For this review, use the dimensioned drawing (mm, ordinates from the lowest corner) and the shaded views. A direction names the side the tool comes from. Coordinates: 2 decimals unless noted, no trailing zeros. Loops run counter-clockwise (first coordinate to the right, second up) from the corner with the lowest first, then second, coordinate; pieces in that order, holes last.
1. Take a section at D-D, the plane y = 65.5. State the section outline as (x, z) points, then the cut area to 3 significant figures.
2. Mouldability with a two-part tool opening along X and no side actions: class the marked faces 1, 2 and 3 as pulls with the +X half, pulls with the -X half, needs draft (parallel to the pull), parting line crosses it, or undercut.
3. Machinability: for the marked faces 4, 5 and 6, which of the approach directions +Z, -Z, +X, -X, +Y, -Y give a long, thin tool a straight path to every point of the face, cutting with its end or side? Answer none if there is none.
4. Take a section at C-C, the plane x = 18. State the section outline as (y, z) points, then the cut area to 4 significant figures.
5. Take a section at A-A, the plane z = 11.5. State the section outline as (x, y) points, then the cut area to 3 significant figures.
6. Take a section at B-B, the plane x = 7.5. State the section outline as (y, z) points.
7. Clearance check with flat-ended pins moving along their axes: P1, Ø15, axis at x = 16.5, y = 123.5, coming from the -Z side; P2, Ø20, axis at x = 16, z = 6.5, coming from the +Y side; P3, Ø10, axis at y = 170.5, z = 44, coming from the -X side; P4, Ø4.5, axis at x = 32, z = 41.5, coming from the -Y side. State where each tip first meets the part, or that it passes through.
8. To check wall thickness, follow probe 1 along Z at (x, y) = (29, 45.5); probe 2 along Y at (x, z) = (18, 7.5); probe 3 along Y at (x, z) = (43, 44). State the ranges of each line that lie inside material, in increasing order.
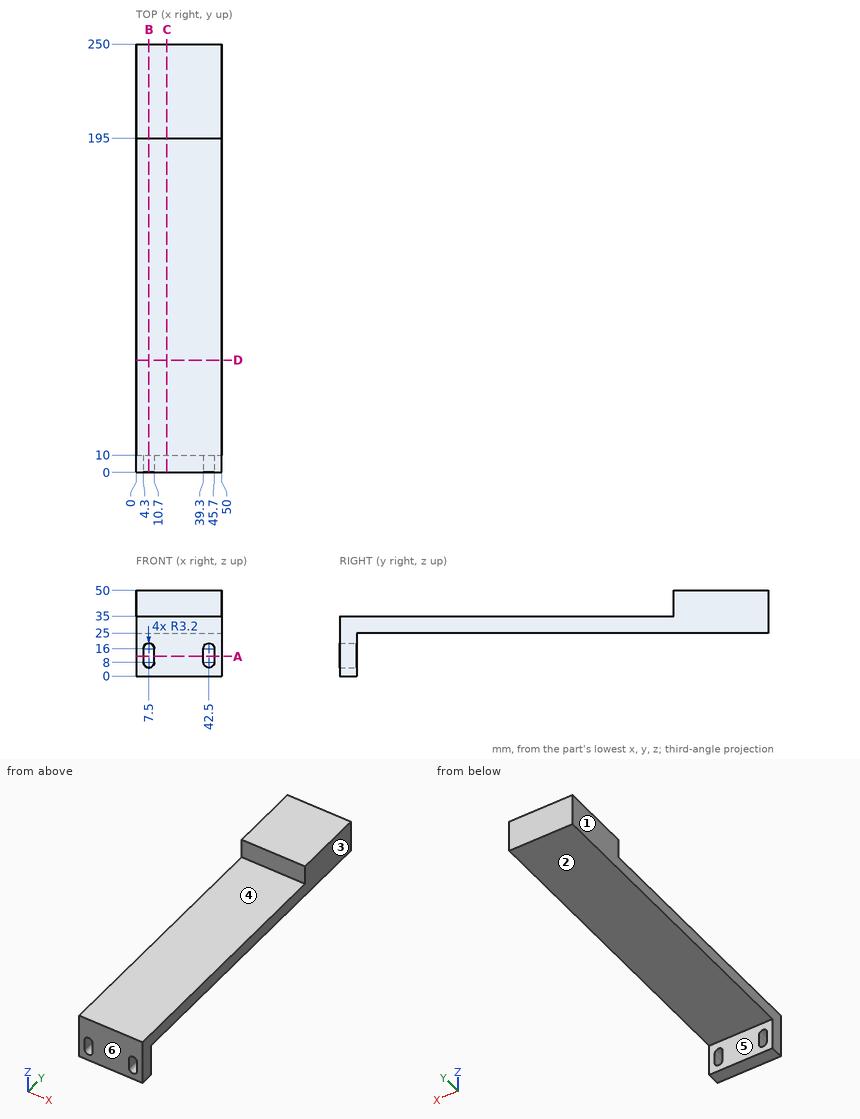
Results list:
1. outline: (0, 25) - (50, 25) - (50, 35) - (0, 35) - close
1. area: 500 mm2
2. face 1: pulls with the -X half
2. face 2: needs draft
2. face 3: pulls with the +X half
3. face 4: +Z, +X, -X, -Y
3. face 5: -Z, +X, -X, +Y
3. face 6: +Z, -Z, +X, -X, -Y
4. outline: (0, 0) - (10, 0) - (10, 25) - (250, 25) - (250, 50) - (195, 50) - (195, 35) - (0, 35) - close
4. area: 3,575 mm2
5. outline: (0, 0) - (4.3, 0) - (4.3, 10) - (0, 10) - close; (10.7, 0) - (39.3, 0) - (39.3, 10) - (10.7, 10) - close; (45.7, 0) - (50, 0) - (50, 10) - (45.7, 10) - close
5. area: 372 mm2
6. outline: (0, 0) - (10, 0) - (10, 4.8) - (0, 4.8) - close; (0, 19.2) - (10, 19.2) - (10, 25) - (250, 25) - (250, 50) - (195, 50) - (195, 35) - (0, 35) - close
7. P1: stops at z = 25
7. P2: stops at y = 10
7. P3: passes through
7. P4: stops at y = 195
8. probe 1: z = 25 to 35
8. probe 2: y = 0 to 10
8. probe 3: y = 195 to 250
